Geometry check sheet. Reference: the model listing, model coordinates, mm. Coordinates: 2 decimals unless noted, no trailing zeros. Order: outer loops, then holes, each group sorted by start corner. A loop starts at its lowest first (then second) coordinate and runs counter-clockwise, first axis right, second up. Notation, with made-up numbers: M -8,-39 L 9,-39 A16 cw 9,-13 Z; hole C -27,45.25 d7. An arc over 180 degrees is marked long. Use CSV: the item, a comma, the result in double quotes. Start each with the question number.
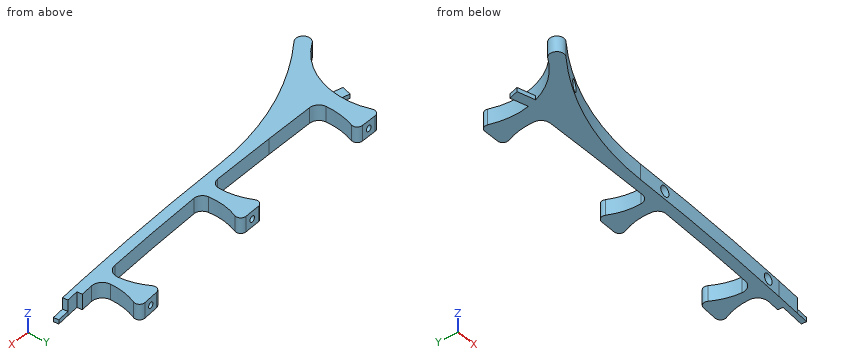
```python
from build123d import *

# Parameters (mm, degrees)
BOSS_EXTRUDE5_START      = -4.7625
BOSS_EXTRUDE5_DEPTH      = 9.525
SKETCH6_R                = 1.778
CUT_EXTRUDE3_DEPTH       = 504.714306696
SKETCH10_R               = 1.778
CUT_EXTRUDE6_DEPTH       = 502.305599176
CUT_EXTRUDE11_DEPTH      = 3.556
CUT_EXTRUDE11_DEPTH_BACK = 499.112065171
SKETCH12_R               = 3.175
SKETCH13_R               = 1.778
CUT_EXTRUDE12_DEPTH      = 500.23676844
CUT_EXTRUDE13_DEPTH      = 6.35
CUT_EXTRUDE13_DEPTH_BACK = 497.697496023
SKETCH14_R               = 3.175
CUT_EXTRUDE14_DEPTH      = 3.556
CUT_EXTRUDE14_DEPTH_BACK = 502.048406711
SKETCH16_R               = 3.175
BOSS_EXTRUDE8_START      = -2.54
BOSS_EXTRUDE8_DEPTH      = 2.54


# Read off the part's stored shape, not the designer's step: Boss-Extrude5
with BuildPart() as part:
    # Boss-Extrude5 outline → Boss-Extrude5 (new body)
    with BuildSketch(Plane(origin=(0, 0, 4.097149242), x_dir=(-1, 0, 0), z_dir=(0, 0, -1)).offset(BOSS_EXTRUDE5_START)):
        with BuildLine():
            add(Edge.make_bspline(
                [(393.904705106, -64.802061588), (391.448326364, -64.761983229), (369.283277897, -64.354767178), (332.573121161, -62.998956248), (298.370755587, -60.752959194), (283.854357877, -59.621991507)],
                knots=[0.399403863, 0.399403863, 0.399403863, 0.399403863, 0.415007942, 0.540214574, 0.632697153, 0.632697153, 0.632697153, 0.632697153], degree=3))
            ThreePointArc((393.904705106, -64.802061588), (443.288872323, -73.243905657), (487.836271638, -96.169655094))
            ThreePointArc((487.836271638, -96.169655094), (494.061542174, -94.986942251), (492.499924864, -88.845757162))
            ThreePointArc((492.499924864, -88.845757162), (472.347982204, -65.669309605), (471.824439099, -34.961421092))
            ThreePointArc((471.824439099, -34.961421092), (471.408544547, -32.082865726), (468.823110549, -30.750731982))
            Line((468.823110549, -30.750731982), (459.298110549, -30.750731982))
            ThreePointArc((459.298110549, -30.750731982), (456.664489609, -32.15241144), (456.356218194, -35.119840174))
            ThreePointArc((456.356218194, -35.119840174), (458.901914687, -43.970050893), (459.537600747, -53.157145299))
            ThreePointArc((459.537600747, -53.157145299), (457.784815205, -57.082003794), (453.798743833, -58.690731982))
            Line((453.798743833, -58.690731982), (423.379813152, -58.69073219))
            add(Edge.make_bspline(
                [(384.460672275, -58.271606449), (385.229576489, -58.288261834), (398.200840977, -58.560856767), (411.17870293, -58.692207634), (423.379813152, -58.69073219)],
                knots=[0.583960389, 0.583960389, 0.583960389, 0.583960389, 0.588862683, 0.666659483, 0.666659483, 0.666659483, 0.666659483], degree=3))
            ThreePointArc((384.460672275, -58.271606449), (381.017085608, -56.831406643), (379.475487665, -53.432003695))
            ThreePointArc((379.475487665, -53.432003695), (380.246820348, -43.884748581), (383.481055682, -34.868942675))
            ThreePointArc((383.481055682, -34.868942675), (383.390574332, -31.793909155), (380.736068027, -30.23904122))
            add(Edge.make_bspline(
                [(371.231646974, -29.984054972), (374.399550345, -30.077611409), (377.567706075, -30.162607104), (380.736068027, -30.23904122)],
                knots=[0.554089987, 0.554089987, 0.554089987, 0.554089987, 0.574612442, 0.574612442, 0.574612442, 0.574612442], degree=3))
            ThreePointArc((371.231646974, -29.984054972), (368.497590279, -31.394357567), (368.242362728, -34.460116711))
            ThreePointArc((368.242362728, -34.460116711), (370.988538335, -43.636366014), (371.246859304, -53.211244668))
            ThreePointArc((371.246859304, -53.211244668), (369.525210394, -56.523100632), (366.009356719, -57.776590868))
            add(Edge.make_bspline(
                [(302.95547422, -54.643284316), (305.9011715, -54.841877501), (317.490683468, -55.594370094), (337.736625716, -56.710847247), (355.814849648, -57.444307809), (365.24066472, -57.751995195), (366.009356719, -57.776590868)],
                knots=[0.410597603, 0.410597603, 0.410597603, 0.410597603, 0.429416671, 0.484628218, 0.539839764, 0.544742054, 0.544742054, 0.544742054, 0.544742054], degree=3))
            ThreePointArc((302.95547422, -54.643284316), (298.577428951, -52.458900104), (297.052141363, -47.809995658))
            ThreePointArc((297.052141363, -47.809995658), (298.741043629, -39.209557534), (302.353410859, -31.223899778))
            ThreePointArc((302.353410859, -31.223899778), (302.446551024, -28.124116994), (299.853176371, -26.423606391))
            add(Edge.make_bspline(
                [(290.370558291, -25.731509235), (293.530799834, -25.970748987), (296.691687874, -26.201449108), (299.853176371, -26.423606391)],
                knots=[0.379296829, 0.379296829, 0.379296829, 0.379296829, 0.399819291, 0.399819291, 0.399819291, 0.399819291], degree=3))
            ThreePointArc((290.370558291, -25.731509235), (287.523350949, -27.0859922), (287.247618484, -30.226881462))
            ThreePointArc((287.247618484, -30.226881462), (289.965925573, -38.51215819), (290.723609817, -47.198982609))
            ThreePointArc((290.723609817, -47.198982609), (288.61383932, -51.750218303), (283.859337385, -53.350089939))
            Line((283.859337385, -53.350089939), (276.361704846, -52.737902091))
            Line((276.361704846, -52.737902091), (276.104683524, -55.885712738))
            Line((276.104683524, -55.885712738), (268.602599978, -55.235621039))
            Line((268.602599978, -55.235621039), (268.333167883, -58.344877914))
            Line((268.333167883, -58.344877914), (283.854357877, -59.621991507))
        make_face()
    extrude(amount=BOSS_EXTRUDE5_DEPTH)

    # Sketch6 → Cut-Extrude3 (cut, through all)
    with BuildSketch(Plane(origin=(0.329495605, -4.514512092, 0), x_dir=(0.9973471252705134, 0.07279225037490757, 0), z_dir=(-0.07279225037490757, 0.9973471252705134, 0))):
        with Locations(Location((-296.227216633, -4.097149242, 0), (0, 0, 180))):
            Circle(SKETCH6_R)
    extrude(amount=-CUT_EXTRUDE3_DEPTH, mode=Mode.SUBTRACT)

    # Sketch10 → Cut-Extrude6 (cut, through all)
    with BuildSketch(Plane(origin=(0.536837, -20.010175041, 0), x_dir=(0.9996403179621594, 0.026818551499160636, 0), z_dir=(-0.026818551499160636, 0.9996403179621594, 0))):
        with Locations(Location((-376.656170964, -4.097149242, 0), (0, 0, 180))):
            Circle(SKETCH10_R)
    extrude(amount=-CUT_EXTRUDE6_DEPTH, mode=Mode.SUBTRACT)

    # Sketch12 → Cut-Extrude11 (cut, two sides: drawn at the far end of the back side and taken through both)
    with BuildSketch(Plane(origin=(1.456593089, -54.293356553, 0), x_dir=(0.9996403179621594, 0.026818551499160636, 0), z_dir=(-0.026818551499160636, 0.9996403179621594, 0)).offset(-CUT_EXTRUDE11_DEPTH_BACK)):
        with Locations(Location((-376.656171029, -4.097149242, 0), (0, 0, 180))):
            Circle(SKETCH12_R)
    extrude(amount=CUT_EXTRUDE11_DEPTH + CUT_EXTRUDE11_DEPTH_BACK, mode=Mode.SUBTRACT)

    # Sketch13 → Cut-Extrude12 (cut, through all)
    with BuildSketch(Plane(origin=(0, -30.750731982, 0), x_dir=(1, 0, 0), z_dir=(0, 1, 0))):
        with Locations(Location((-464.060610549, -4.097149242, 0), (0, 0, 270))):
            Circle(SKETCH13_R)
    extrude(amount=-CUT_EXTRUDE12_DEPTH, mode=Mode.SUBTRACT)

    # Sketch14 → Cut-Extrude13 (cut, two sides: drawn at the far end of the back side and taken through both)
    with BuildSketch(Plane(origin=(0, -68.850731982, 0), x_dir=(1, 0, 0), z_dir=(0, 1, 0)).offset(-CUT_EXTRUDE13_DEPTH_BACK)):
        with Locations(Location((-464.060610549, -4.097149242, 0), (0, 0, 270))):
            Circle(SKETCH14_R)
    extrude(amount=CUT_EXTRUDE13_DEPTH + CUT_EXTRUDE13_DEPTH_BACK, mode=Mode.SUBTRACT)

    # Sketch16 → Cut-Extrude14 (cut, two sides: drawn at the far end of the back side and taken through both)
    with BuildSketch(Plane(origin=(2.82554187, -38.713545018, 0), x_dir=(0.9973471252705134, 0.07279225037490757, 0), z_dir=(-0.07279225037490757, 0.9973471252705134, 0)).offset(-CUT_EXTRUDE14_DEPTH_BACK)):
        with Locations(Location((-296.227216633, -4.097149242, 0), (0, 0, 180))):
            Circle(SKETCH16_R)
    extrude(amount=CUT_EXTRUDE14_DEPTH + CUT_EXTRUDE14_DEPTH_BACK, mode=Mode.SUBTRACT)

    # Sketch17 → Boss-Extrude8 (add)
    with BuildSketch(Plane(origin=(0, 0, -0.665350758), x_dir=(-1, 0, 0), z_dir=(0, 0, -1)).offset(BOSS_EXTRUDE8_START)):
        Polygon((480.741163163, -55.807148253), (482.353687842, -61.5964138), (471.918866371, -64.502897707), (470.306341692, -58.71363216), align=None)
        Polygon((268.602599978, -55.235621039), (260.960708561, -54.573414315), (260.691276466, -57.68267119), (268.333167883, -58.344877914), align=None)
        with BuildLine():
            ThreePointArc((471.918866371, -64.502897707), (471.01556343, -61.635294332), (470.306341692, -58.71363216))
            Line((470.306341692, -58.71363216), (468.875088895, -59.112289025))
            Line((468.875088895, -59.112289025), (470.487613574, -64.901554572))
            Line((470.487613574, -64.901554572), (471.918866371, -64.502897707))
        make_face()
        with BuildLine():
            Line((471.918866371, -64.502897707), (470.306341692, -58.71363216))
            ThreePointArc((470.306341692, -58.71363216), (471.01556343, -61.635294332), (471.918866371, -64.502897707))
        make_face()
    extrude(amount=BOSS_EXTRUDE8_DEPTH)


solid = part.part
```
1) Section check C-C on y = -92. Record the boundary of the cut face in (x, z), then the cut area to 3 significant figures.
2) Gauge pin test, flat ends, axial feed: P1, Ø3, axis at x = -437, z = 6, coming from the +Y side; P2, Ø3, axis at x = -463, z = 3, coming from the -Y side; P3, Ø9.5, axis at x = -476, y = -61, coming from the +Z side; P4, Ø3, axis at x = -464.06, z = 4.1, coming from the +Y side. Record the tip position at first contact, or that the pin passes through.
3) Section check D-D on x = -429.5. Record the boundary of the cut face in (y, z), then the cut area to 3 significant figures.
4) Material ranges on line 1 along X through (y, z) = (-33.5, 6); line 2 along X through (y, z) = (-45, 6); line 3 along X through (y, z) = (-30.5, 2.25), recorded low to high.
5) Section check A-A on x = -475.5. Record the boundary of the cut face in (y, z), then the cut area to 3 significant figures.
6) Section check B-B on y = -74. Record the boundary of the cut face in (x, z) (3 decimals).
Results are:
1,outline,"M -494.69,-0.67 L -481.82,-0.67 L -481.82,8.86 L -494.69,8.86 Z"
1,area,"123 mm²"
2,P1,"stops at y = -58.69"
2,P2,"stops at y = -62.5"
2,P3,"stops at z = 1.87"
2,P4,"passes through"
3,outline,"M -69.3,-0.67 L -58.69,-0.67 L -58.69,8.86 L -69.3,8.86 Z"
3,area,"101 mm²"
4,line 1,"x = -471.97 to -456.15, -383.83 to -367.98, -301.09 to -288.58"
4,line 2,"x = -469.61 to -459.07, -380.02 to -371.18, -297.38 to -290.72"
4,line 3,"x = -381.92 to -369.4, -302.67 to -287.37"
5,outline,"M -88.03,-0.67 L -72.23,-0.67 L -72.23,8.86 L -88.03,8.86 Z; M -63.51,-0.67 L -57.27,-0.67 L -57.27,1.87 L -63.51,1.87 Z"
5,area,"166 mm²"
6,outline,"M -476.587,-0.665 L -445.501,-0.665 L -445.501,8.86 L -476.587,8.86 Z; hole C -464.061,4.097 d6.35"
